For this review, use the dimensioned drawing (mm, ordinates from the lowest corner) and the shaded views. A direction names the side the tool comes from. Give positions to 0.01 mm unless a question says otherwise; leave off trailing zeros. Write each loop counter-clockwise with the first axis right and the second up, starting at its lowest first coordinate (ties: lowest second). Pieces come first, ordered by that corner, then holes.
1) Wall thickness on line 1 along Z through (x, y) = (11, 7); line 2 along X through (y, z) = (0.5, 158.5); line 3 along Y through (x, z) = (8, 96): over which ranges is each line inside the solid? List them lowest first.
2) We need section B-B on z = 25.5. Give the boundary of the cut face in (x, y), and give its area (3 significant figures).
3) We need section C-C on y = 11.25. Give the boundary of the cut face in (x, z), and give its area (3 significant figures).
4) We need section A-A on x = 13. Give the boundary of the cut face in (y, z).
5) For P1, Ø5, axis at x = 18.5, z = 149, coming from the -Y side; P2, Ø2.5, axis at x = 13.5, y = 8, coming from the -Z side; P3, Ø1.5, axis at y = 5.5, z = 38.5, coming from the +X side, all flat-tipped, find the tip position at first contact; note any pin that passes through.
6) We need section D-D on z = 111.5. Give the boundary of the cut face in (x, y), and give its area (3 significant figures).
7) Machinability: for the marked faces 1 and 2, which of the approach directions +Z, -Z, +X, -X, +Y, -Y give a long, thin tool a straight path to every point of the face, cutting with its end or side? Answer none if there is none.
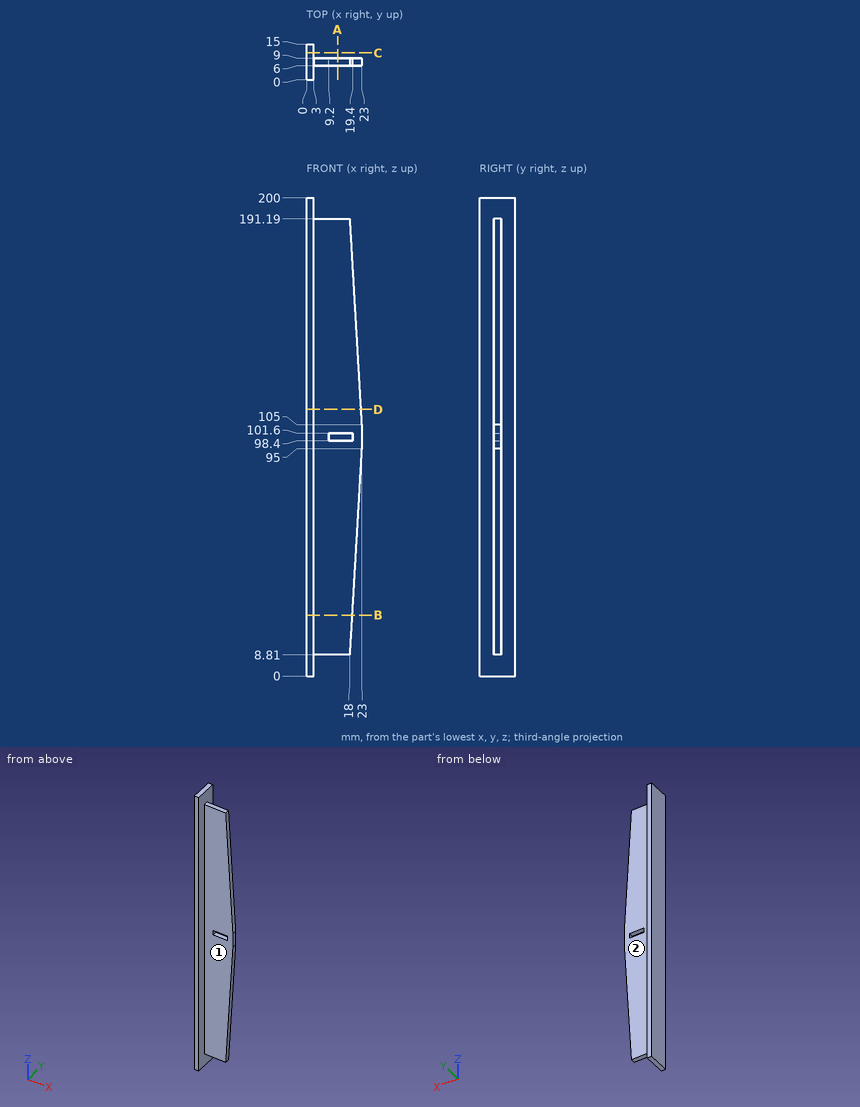
Results list:
1. line 1: z = 8.81 to 98.4, 101.6 to 191.19
1. line 2: x = 0 to 3
1. line 3: y = 6 to 9
2. outline: (0, 0) - (3, 0) - (3, 6) - (18.97, 6) - (18.97, 9) - (3, 9) - (3, 15) - (0, 15) - close
2. area: 92.9 mm2
3. outline: (0, 0) - (3, 0) - (3, 200) - (0, 200) - close
3. area: 600 mm2
4. outline: (6, 8.81) - (9, 8.81) - (9, 98.4) - (6, 98.4) - close; (6, 101.6) - (9, 101.6) - (9, 191.19) - (6, 191.19) - close
5. P1: stops at y = 6
5. P2: stops at z = 8.81
5. P3: stops at x = 19.75
6. outline: (0, 0) - (3, 0) - (3, 6) - (22.62, 6) - (22.62, 9) - (3, 9) - (3, 15) - (0, 15) - close
6. area: 104 mm2
7. face 1: +Z, -Z, +X, -Y
7. face 2: +Z, -Z, +X, +Y
